Autodesk Inventor part; units mm, degrees
ref_plane "Start plane" through (0, 0, 0) normal (0, 0, 1) x (1, 0, 0)
ref_plane "End plane" through (0, 0, 406.4) normal (0, 0, 1) x (1, 0, 0)
ref_plane "Work Plane4" through (444.5, 0, 0) normal (-1, 0, 0) x (0, 0, 1)
ref_plane "Start plane" through (0, 0, 0) normal (0, 0, 1) x (1, 0, 0)
ref_plane "End plane" through (0, 0, 406.4) normal (0, 0, 1) x (1, 0, 0)
sketch "Sketch" plane through (0, 0, 0) normal (0, 0, 1) x (1, 0, 0)
  circle A0 centre (0, 0) radius 13.3223
  circle A1 centre (0, 0) radius 16.7005
  dimension "d0" = 33.401
  dimension "d1" = 3.3782
extrude "Body" add sketch "Sketch" along normal up to surface (406.4 mm away) from surface at 0
sketch "Sketch3" plane through (0, 0, 0) normal (0, 0, 1) x (1, 0, 0)
  line L0 (0, 0) -> (10, 0)
ref_plane "Work Plane3" through (0, 0, 0) normal (0, -1, 0) x (1, 0, 0)
sketch "Sketch4" plane through (0, 0, 0) normal (0, -1, 0) x (1, 0, 0)
  line L0 (-2, 0) -> (12, 0)
  line L1 (-2, 406.4) -> (12, 406.4)
  dimension "d7" = 406.4
ref_plane "Work Plane4" through (444.5, 0, 0) normal (-1, 0, 0) x (0, 0, 1)
ref_plane "Work Plane5" through (-355.6, 0, 0) normal (-1, 0, 0) x (0, 0, 1)
ref_plane "Work Plane6" through (44.45, 0, 0) normal (-1, 0, 0) x (0, 0, 1)
sketch "Sketch5" plane through (44.45, 0, 0) normal (-1, 0, 0) x (0, 0, 1)
  circle A0 centre (0, 0) radius 16.7005
  circle A1 centre (0, 0) radius 13.3223
extrude "Extrusion2" cut sketch "Sketch5" along normal up to surface (800.1 mm away) from surface at -400.05 contours A0 | A1
ref_plane "Work Plane7" through (-355.6, 0, 406.4) normal (1, 0, 0) x (0, 0, -1)
ref_plane "Work Plane8" through (444.5, 0, 406.4) normal (1, 0, 0) x (0, 0, -1)
ref_plane "Work Plane9" through (44.45, 0, 406.4) normal (1, 0, 0) x (0, 0, -1)
sketch "Sketch6" plane through (44.45, 0, 406.4) normal (1, 0, 0) x (0, 0, -1)
  circle A0 centre (0, 0) radius 16.7005
  circle A1 centre (0, 0) radius 13.3223
extrude "Extrusion3" cut sketch "Sketch6" along normal up to surface (800.1 mm away) from surface at -400.05 contours A0 | A1
equation "\"d0\" = G_H"
equation "\"d1\" = G_T"
equation "\"d2\" = G_L"
equation "\"G_H\" = 33.401"
equation "\"G_T\" = 3.3782"
equation "\"G_L\" = d7"
equation "\"G_OFFSET_START\" = 0"
equation "\"G_OFFSET_END\" = 0"
equation "\"d5\" = G_OFFSET_END + B_L"
equation "\"B_L\" = 406.4"
properties part number "ANSI - 1 x 0.133 - 16" material "Aluminum 6061"
Here's how the part is built. I have some questions about the finished solid (model axes, mm). Coordinates: 2 decimals unless noted, no trailing zeros. Order: outer loops, then holes, each group sorted by start corner. A loop starts at its lowest first (then second) coordinate and runs counter-clockwise, first axis right, second up. Notation, with made-up numbers: (66.5, 45) - (81.5, 45) arc R28 cw to (81.5, 72) - close; hole circle Ø5 at (15.5, 3). An arc over 180 degrees is marked (long way). One line per question, with ' | ' between items. Start each with the question number.
1. If we section it at B-B (x = 0): Write out the boundary of the cut face in (y, z).
2. Please list where these lines run through material, in increasing order: line 1 along Y through (x, z) = (0, 260); line 2 along X through (y, z) = (-6, 208). Write a range as [from, to].
3. I'm going to push flat-ended pins straight in: pin 1 Ø1 at (y, z) = (-11.5, 166) entering from +X; pin 2 Ø4 at (x, z) = (7, 135) entering from +Y; pin 3 Ø1 at (x, z) = (-3, 138.5) entering from +Y; pin 4 Ø16 at (x, y) = (0, 0) entering from -Z. Where does each tip first touch, or does it pass through?
4. If we section it at C-C (z = 191): Write out the boundary of the cut face in (x, y), and give its area (3 significant figures).
5. If we mould it in two halves opening along Y, with no side actions, what happens to faces 1 (the cylindrical face through (12.707, -4.002, 200.496)), 2 (the cylindrical face through (-3.62, 16.303, 200.355))? For each: released by +Y, released by -Y, zero draft, split by the parting line, or undercut.
6. If we section it at A-A (y = 0): Write out the boundary of the cut face in (x, z), and give its area (3 significant figures).
Model answer:
1) outline: (-16.7, 0) arc R16.7 cw to (-13.32, 10.07) - (-13.32, 396.33) arc R16.7 cw to (-16.7, 406.4) - close; (13.32, 10.07) arc R16.7 cw to (16.7, 0) - (16.7, 406.4) arc R16.7 cw to (13.32, 396.33) - close
2) line 1: y = [-16.7, -13.32], [13.32, 16.7] | line 2: x = [-15.59, -11.89], [11.89, 15.59]
3) pin 1: stops at x = 12.57 | pin 2: stops at y = 15.93 | pin 3: stops at y = 16.51 | pin 4: passes through
4) outline: circle Ø33.4 at (0, 0); hole circle Ø26.64 at (0, 0) | area: 319 mm²
5) face 1: undercut | face 2: split by the parting line
6) outline: (-16.7, 16.7) - (-13.32, 16.7) - (-13.32, 389.7) - (-16.7, 389.7) - close; (13.32, 16.7) - (16.7, 16.7) - (16.7, 389.7) - (13.32, 389.7) - close | area: 2,520 mm²
